```python
from build123d import *

# Parameters (mm, degrees)
SKETCH1_R           = 12
BOSS_EXTRUDE1_DEPTH = 5
SKETCH2_R           = 6.5
BOSS_EXTRUDE2_DEPTH = 4
SKETCH3_R           = 5.1
CUT_EXTRUDE1_DEPTH  = 7
SKETCH4_R           = 4
CUT_EXTRUDE2_DEPTH  = 7


with BuildPart() as part:
    # Sketch1 → Boss-Extrude1 (new body)
    with BuildSketch(Plane(origin=(0, 0, 0), x_dir=(1, 0, 0), z_dir=(0, 1, 0))):
        Circle(SKETCH1_R)
    extrude(amount=BOSS_EXTRUDE1_DEPTH)

    # Sketch2 → Boss-Extrude2 (add)
    with BuildSketch(Plane(origin=(0, 5, 0), x_dir=(1, 0, 0), z_dir=(0, 1, 0))):
        Circle(SKETCH2_R)
    extrude(amount=BOSS_EXTRUDE2_DEPTH)

    # Sketch3 → Cut-Extrude1 (cut)
    with BuildSketch(Plane.XZ):
        Circle(SKETCH3_R)
    extrude(amount=-CUT_EXTRUDE1_DEPTH, mode=Mode.SUBTRACT)

    # Sketch4 → Cut-Extrude2 (cut)
    with BuildSketch(Plane(origin=(0, 9, 0), x_dir=(1, 0, 0), z_dir=(0, 1, 0))):
        Circle(SKETCH4_R)
    extrude(amount=-CUT_EXTRUDE2_DEPTH, mode=Mode.SUBTRACT)


solid = part.part
```
Could you check a few things on this model? Use its own coordinates, in mm. A direction names the side the tool comes from. Round coordinates to 2 decimals unless told otherwise and drop trailing zeros. Loops run counter-clockwise (first coordinate to the right, second up) from the corner with the lowest first, then second, coordinate; pieces in that order, holes last.
Q1. I want a section at D-D (z = 4.5). Write out the boundary of the cut face in (x, y).
Q2. On a 3-axis mill with a long thin cutter (end or side, diameter ignored), from which of +Z, -Z, +X, -X, +Y, -Y can I reach the whole of each face in a straight line? I mean faces 1 (the cylindrical face through (2.4, 3.5, -4.5)), 2 (the cylindrical face through (-5.158, 6.972, 3.955)), 3 (the flat face through (5, 0, 2)). Say none if no direction works.
Q3. I want a section at C-C (y = 3.25). Write out the boundary of the cut face in (x, z), and give its area (3 significant figures).
Q4. Thinking about a two-plate mould opening in X: for faces 4 (the cylindrical face through (-11.99, 2.46, -0.53)), 5 (the flat face through (5, 5, 5)), 6 (the flat face through (-3, 7, -3)), 7 (the cylindrical face through (-0.867, 8.014, 3.905)), which applies, pulls with the +X half, pulls with the -X half, needs draft (parallel to the pull), parting line crosses it, or undercut?
Q5. For P1, Ø6, axis at x = -3.5, z = -9, coming from the +Y side; P2, Ø1, axis at x = -3, y = 8, coming from the -Z side, each with a flat end and sliding along its axis, tell me the tip position at first contact or that it passes through.
Q6. I want a section at B-B (z = 0). Write out the boundary of the cut face in (x, y), and give its area (3 significant figures).
Q7. I want a section at A-A (x = 0). Write out the boundary of the cut face in (y, z), and give its area (3 significant figures).
Q8. Please list where these lines run through material, in increasing order: L1, parallel to Z at x = 0, y = 7.5; L2, parallel to Y at x = -10, z = 3.25.
Answer below:
1. outline: (-11.12, 0) - (-2.4, 0) - (-2.4, 7) - (2.4, 7) - (2.4, 0) - (11.12, 0) - (11.12, 5) - (4.69, 5) - (4.69, 9) - (-4.69, 9) - (-4.69, 5) - (-11.12, 5) - close
2. face 1: -Y
2. face 2: +Y
2. face 3: +Z, -Z, +X, -X, -Y
3. outline: circle Ø24 at (0, 0); hole circle Ø10.2 at (0, 0)
3. area: 371 mm2
4. face 4: parting line crosses it
4. face 5: needs draft
4. face 6: undercut
4. face 7: undercut
5. P1: stops at y = 5
5. P2: stops at z = -6
6. outline: (-12, 0) - (-5.1, 0) - (-5.1, 7) - (-4, 7) - (-4, 9) - (-6.5, 9) - (-6.5, 5) - (-12, 5) - close; (4, 7) - (5.1, 7) - (5.1, 0) - (12, 0) - (12, 5) - (6.5, 5) - (6.5, 9) - (4, 9) - close
6. area: 84.6 mm2
7. outline: (0, -12) - (5, -12) - (5, -6.5) - (9, -6.5) - (9, -4) - (7, -4) - (7, -5.1) - (0, -5.1) - close; (0, 5.1) - (7, 5.1) - (7, 4) - (9, 4) - (9, 6.5) - (5, 6.5) - (5, 12) - (0, 12) - close
7. area: 84.6 mm2
8. L1: z = -6.5 to -4, 4 to 6.5
8. L2: y = 0 to 5
